Input: part model. Units: mm. Frame: model coordinates. Face numbers are marked on the shaded views. A direction names the side the tool comes from. Coordinates: 2 decimals unless noted, no trailing zeros. Loops run counter-clockwise (first coordinate to the right, second up) from the corner with the lowest first, then second, coordinate; pieces in that order, holes last. Notation, with made-up numbers: (-8, -34.75) -> (43, -34.75) arc R20 cw to (43, -7.75) -> close; hole circle Ø5 at (43, -37). An arc over 180 degrees is marked (long way). Put each result on its own line as item: value. Start each with the question number.
1) Cut plane A-A (y = 13). Return the cut outline in (x, z), plus the area to 3 significant figures.
2) Set-up query: the marked faces 1 and 2. Return all of +Z, -Z, +X, -X, +Y, -Y with unobstructed straight access to the full face (end or side cutting, diameter ignored); none if empty.
3) Cut plane B-B (y = -28). Return the cut outline in (x, z).
4) Material intervals for L1, parallel to Z at x = 18, y = -27; L2, parallel to X at y = -3.5, z = 0.25; L3, parallel to Z at x = 3, y = -22, sorted ascending.
5) Contact query for flat-ended pins moving along their axis: P1, Ø1.3, axis at y = -25.5, z = -12, coming from the +X side; P2, Ø0.6, axis at y = -25, z = -12, coming from the -X side; P3, Ø2, axis at x = 39.5, z = -16, coming from the -Y side. Output: stop coordinate, or through.
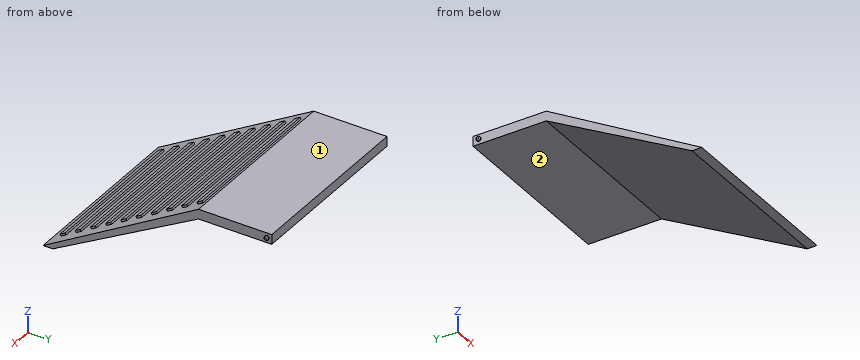
from build123d import *

# Parameters (mm, degrees)
F0_W     = 19.05
F0_H     = 2.54
F1_DEPTH = 46.99
F2_W     = 40.0845290253
F2_H     = 1.524
F3_DEPTH = 0.508
F4_R     = 0.57150051
F5_DEPTH = 0.508
F6_R     = 0.254
F7_R     = 0.5715
F8_DEPTH = 0.508
F9_R     = 0.254


with BuildPart() as f1:
    # F0 (on Right) → F1 (new body)
    with BuildSketch(Plane.YZ):
        with Locations((9.525, 1.27)):
            Rectangle(F0_W, F0_H)
        Polygon((0, 0), (0, 2.54), (-40.4138714075, -20.9532231092), (-37.8738714075, -20.9532231092), align=None)
    extrude(amount=F1_DEPTH)

    # F2 (on face) → F3 (join)
    with BuildSketch(Plane(origin=(0, -1.1036035582, 1.8984577841), x_dir=(1, 0, 0), z_dir=(0, -0.5025690754, 0.8645370579))):
        with Locations((23.495, -0.7067697006)):
            Rectangle(F2_W, F2_H)
        with Locations((23.495, -5.2787697006)):
            Rectangle(F2_W, F2_H)
        with Locations((23.495, -9.8507697006)):
            Rectangle(F2_W, F2_H)
        with Locations((23.495, -14.4227697006)):
            Rectangle(F2_W, F2_H)
        with Locations((23.495, -18.9947697006)):
            Rectangle(F2_W, F2_H)
        with Locations((23.495, -23.5667697006)):
            Rectangle(F2_W, F2_H)
        with Locations((23.495, -28.1387697006)):
            Rectangle(F2_W, F2_H)
        with Locations((23.495, -32.7107697006)):
            Rectangle(F2_W, F2_H)
        with Locations((23.495, -37.2827697006)):
            Rectangle(F2_W, F2_H)
        with Locations((23.495, -41.8547697006)):
            Rectangle(F2_W, F2_H)
    extrude(amount=F3_DEPTH)

    # F4 (on face) → F5 (join)
    with BuildSketch(Plane(origin=(0, 0, 0), x_dir=(0, -1, 0), z_dir=(-1, 0, 0))):
        with Locations((-17.5560880452, 1.3172084)):
            Circle(F4_R)
    extrude(amount=F5_DEPTH)

    # F6
    f6_edges = [f1.edges().sort_by_distance(p)[0] for p in [
        (-0.508, 18.127589, 1.317208),
    ]]
    fillet(f6_edges, radius=F6_R)

    # F7 (on face) → F8 (join)
    with BuildSketch(Plane.YZ.offset(46.99)):
        with Locations((17.8131051362, 1.299622003)):
            Circle(F7_R)
    extrude(amount=F8_DEPTH)

    # F9
    f9_edges = [f1.edges().sort_by_distance(p)[0] for p in [
        (47.498, 17.241605, 1.299622),
    ]]
    fillet(f9_edges, radius=F9_R)


solid = f1.part
Results found:
1. outline: (0, 0) -> (46.99, 0) -> (46.99, 2.54) -> (0, 2.54) -> close
1. area: 119 mm2
2. face 1: +Z, +X, -X, +Y, -Y
2. face 2: -Z, +X, -X, +Y
3. outline: (0, -15.49) -> (46.99, -15.49) -> (46.99, -13.74) -> (0, -13.74) -> close
4. L1: z = -14.94 to -13.16
4. L2: x = 0 to 46.99
4. L3: z = -12.17 to -10.25
5. P1: stops at x = 46.99
5. P2: stops at x = 0
5. P3: stops at y = -34.25
